The listing builds one solid part. Answer for the finished solid, in the listing's coordinates (mm). A direction names the side the tool comes from. Give positions to 0.01 mm unless a question says otherwise; leave off trailing zeros. Write each loop counter-clockwise with the first axis right and the second up, starting at its lowest first coordinate (ties: lowest second). Pieces come first, ordered by that corner, then holes. Notation, with made-up numbers: (15, 89) - (69, 89) arc R33 cw to (69, 117) - close; hole circle Ø1 at (-17, -39). An arc over 180 degrees is marked (long way). Return JSON: item names as keys, results as strings.
from build123d import *

# Parameters (mm, degrees)
F2_DEPTH = 2


with BuildPart() as f2:
    # F1 (on Top) → F2 (new body)
    with BuildSketch(Plane.XY):
        Polygon((17.7639320225, 10), (-17.7639320225, 10), (-13.7639320225, 8), (13.7639320225, 8), align=None)
        Polygon((10.7639320225, 6.5), (-10.7639320225, 6.5), (-6.7639320225, 4.5), (6.7639320225, 4.5), align=None)
        Polygon((-18, 7.8819660113), (-20, 8.8819660113), (-20, -8.8819660113), (-18, -7.8819660113), align=None)
        Polygon((-11, 4.3819660113), (-13, 5.3819660113), (-13, -5.3819660113), (-11, -4.3819660113), align=None)
        Polygon((-2.2360679775, 0), (-11, -4.3819660113), (-11, -4.5), (-6.7639320225, -4.5), (0, -1.1180339887), align=None)
        Polygon((20, -8.8819660113), (20, 8.8819660113), (18, 7.8819660113), (18, -7.8819660113), align=None)
        Polygon((11, -4.3819660113), (2.2360679775, 0), (0, -1.1180339887), (6.7639320225, -4.5), (11, -4.5), align=None)
        Polygon((11, 4.5), (6.7639320225, 4.5), (0, 1.1180339887), (2.2360679775, 0), (11, 4.3819660113), align=None)
        Polygon((-17.7639320225, 10), (-20, 10), (-20, 8.8819660113), (-18, 7.8819660113), (-18, 8), (-13.7639320225, 8), align=None)
        Polygon((-10.7639320225, 6.5), (-13.7639320225, 8), (-18, 8), (-18, 7.8819660113), (-13, 5.3819660113), (-13, 6.5), align=None)
        Polygon((-6.7639320225, 4.5), (-10.7639320225, 6.5), (-13, 6.5), (-13, 5.3819660113), (-11, 4.3819660113), (-11, 4.5), align=None)
        Polygon((20, 10), (17.7639320225, 10), (13.7639320225, 8), (18, 8), (18, 7.8819660113), (20, 8.8819660113), align=None)
        Polygon((18, 8), (13.7639320225, 8), (10.7639320225, 6.5), (13, 6.5), (13, 5.3819660113), (18, 7.8819660113), align=None)
        Polygon((13, 6.5), (10.7639320225, 6.5), (6.7639320225, 4.5), (11, 4.5), (11, 4.3819660113), (13, 5.3819660113), align=None)
        Polygon((2.2360679775, 0), (0, 1.1180339887), (-2.2360679775, 0), (0, -1.1180339887), align=None)
        Polygon((0, 1.1180339887), (-6.7639320225, 4.5), (-11, 4.5), (-11, 4.3819660113), (-2.2360679775, 0), align=None)
        Polygon((-11, -4.3819660113), (-13, -5.3819660113), (-13, -6.5), (-10.7639320225, -6.5), (-6.7639320225, -4.5), (-11, -4.5), align=None)
        Polygon((-13, -5.3819660113), (-18, -7.8819660113), (-18, -8), (-13.7639320225, -8), (-10.7639320225, -6.5), (-13, -6.5), align=None)
        Polygon((-18, -7.8819660113), (-20, -8.8819660113), (-20, -10), (-17.7639320225, -10), (-13.7639320225, -8), (-18, -8), align=None)
        Polygon((-13.7639320225, -8), (-17.7639320225, -10), (17.7639320225, -10), (13.7639320225, -8), align=None)
        Polygon((20, -10), (20, -8.8819660113), (18, -7.8819660113), (18, -8), (13.7639320225, -8), (17.7639320225, -10), align=None)
        Polygon((18, -8), (18, -7.8819660113), (13, -5.3819660113), (13, -6.5), (10.7639320225, -6.5), (13.7639320225, -8), align=None)
        Polygon((13, -6.5), (13, -5.3819660113), (11, -4.3819660113), (11, -4.5), (6.7639320225, -4.5), (10.7639320225, -6.5), align=None)
        Polygon((-6.7639320225, -4.5), (-10.7639320225, -6.5), (10.7639320225, -6.5), (6.7639320225, -4.5), align=None)
        Polygon((13, -5.3819660113), (13, 5.3819660113), (11, 4.3819660113), (11, -4.3819660113), align=None)
    extrude(amount=F2_DEPTH)


solid = f2.part
Item 1: Consider L1, parallel to X at y = -5, z = 1.7; L2, parallel to Y at x = 0, z = 0.25; L3, parallel to Y at x = 9, z = 1.5. Determine where each line is inside the solid, lowest interval first.
Answer below:
{"L1": "x = -20 to -18, -13 to 13, 18 to 20", "L2": "y = -10 to -8, -6.5 to -4.5, -1.12 to 1.12, 4.5 to 6.5, 8 to 10", "L3": "y = -10 to -8, -6.5 to -3.38, 3.38 to 6.5, 8 to 10"}
Item 2: A cutting plane is placed at A-A on y = -5. Determine the outline of the cut face in (x, z).
Answer below:
{"outline": "(-20, 0) - (-18, 0) - (-18, 2) - (-20, 2) - close; (-13, 0) - (13, 0) - (13, 2) - (-13, 2) - close; (18, 0) - (20, 0) - (20, 2) - (18, 2) - close"}
Item 3: For faces 5 (the face through (-15.54, 6.65, 0.99)), 6 (the face through (-5, 2, 0)), determine the directions among +Z, -Z, +X, -X, +Y, -Y from which every point of the face is accessible in a straight line to the end or side of a thin tool.
Answer below:
{"face 5": "+Z, -Z", "face 6": "-Z, +X, -X, +Y, -Y"}
Item 4: A cutting plane is placed at B-B on z = 1.1. Give the number of separate pieces and of enclosed holes in the cut face, then the cut area to 3 significant figures.
Answer below:
{"separate pieces": "1", "enclosed holes": "8", "area": "471 mm²"}
Item 5: The mould has two halves that part along X. Classify faces 1 (the face through (3.429, 2.833, 0.986)), 2 (the face through (20, 0, 1)), 3 (the face through (-5, 2, 2)), 4 (the face through (0, 4.5, 1)): +X half, -X half, draft (parallel to the pull), parting line (faces both ways), or undercut.
Answer below:
{"face 1": "undercut", "face 2": "+X half", "face 3": "draft", "face 4": "undercut"}
Item 6: A cutting plane is placed at C-C on x = -1. Determine the outline of the cut face in (y, z).
Answer below:
{"outline": "(-10, 0) - (-8, 0) - (-8, 2) - (-10, 2) - close; (-6.5, 0) - (-4.5, 0) - (-4.5, 2) - (-6.5, 2) - close; (-1.62, 0) - (1.62, 0) - (1.62, 2) - (-1.62, 2) - close; (4.5, 0) - (6.5, 0) - (6.5, 2) - (4.5, 2) - close; (8, 0) - (10, 0) - (10, 2) - (8, 2) - close"}
Item 7: A cutting plane is placed at D-D on y = -7.5. Determine the outline of the cut face in (x, z), then the cut area to 3 significant figures.
Answer below:
{"outline": "(-20, 0) - (-18, 0) - (-18, 2) - (-20, 2) - close; (-17.24, 0) - (-12.76, 0) - (-12.76, 2) - (-17.24, 2) - close; (12.76, 0) - (17.24, 0) - (17.24, 2) - (12.76, 2) - close; (18, 0) - (20, 0) - (20, 2) - (18, 2) - close", "area": "25.9 mm²"}
